Work out the finished part from the listing and answer in its coordinate system (mm). Face numbers are marked on the shaded views. Give positions to 0.01 mm unless a question says otherwise; leave off trailing zeros. Write each loop counter-clockwise with the first axis right and the second up, starting at its lowest first coordinate (ties: lowest second). Pieces come first, ordered by that corner, then holes. Notation, with made-up numbers: (77.5, 14) - (136.5, 14) arc R34 cw to (136.5, 47) - close; hole circle Ø5 at (-16.5, 5). An arc over 180 degrees is marked (long way). Write item = value, one per line.
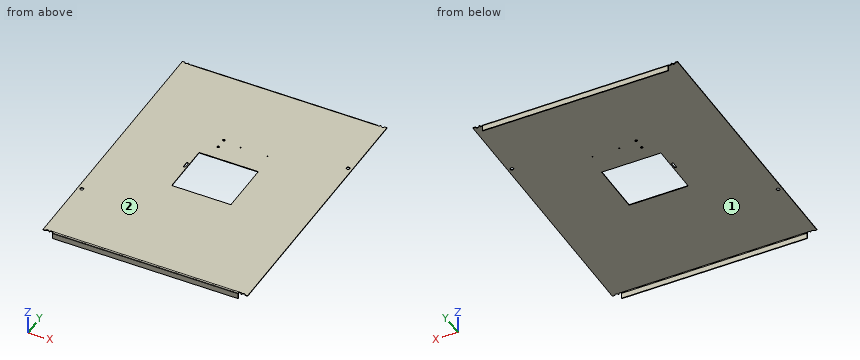
from build123d import *

# Parameters (mm, degrees)
CROQUIS1_W                   = 482.6
CROQUIS1_H                   = 634.238
BRIDA_BASE1_DEPTH            = 1.524
CROQUIS6_R                   = 3.9624
CROQUIS6_W                   = 6.35
CROQUIS6_H                   = 3.048
CORTAR_EXTRUIR1_DEPTH        = 399.487732229
BRIDA_START                  = -218.948
BRIDA_DE_ARISTA1_DEPTH       = 437.896
BRIDA_START_2                = -219.1004
BRIDA_DE_ARISTA1_2_OUTLINE_W = 0.1524
BRIDA_DE_ARISTA1_2_OUTLINE_H = 1.524
BRIDA_DE_ARISTA1_2_DEPTH     = 0.1524
BRIDA_START_3                = 218.948
BRIDA_DE_ARISTA1_3_OUTLINE_W = 0.1524
BRIDA_DE_ARISTA1_3_OUTLINE_H = 1.524
BRIDA_DE_ARISTA1_3_DEPTH     = 0.1524
BRIDA_DE_ARISTA1_4_DEPTH     = 437.896
CORTAR_EXTRUIR2_REACH        = 400.806
CROQUIS13_R                  = 3.9624
CROQUIS13_R_2                = 2.8956
CROQUIS13_R_3                = 1.27
CROQUIS13_W                  = 139.7
CROQUIS13_H                  = 124.714
CROQUIS13_W_2                = 4.826
CROQUIS13_H_2                = 16.002


# Read off the part's stored shape, not the designer's step: Brida de arista1
# Sheet-metal steps are written as plain solids
with BuildPart() as part:
    # Croquis1 → Brida base1 (new body)
    with BuildSketch(Plane.XY):
        Rectangle(CROQUIS1_W, CROQUIS1_H)
    extrude(amount=-BRIDA_BASE1_DEPTH)

    # Croquis6 → Cortar-Extruir1 (cut, through all)
    with BuildSketch(Plane.XY):
        with Locations((231.648, 317.627)):
            Circle(CROQUIS6_R)
        with Locations((-231.648, 317.627)):
            Circle(CROQUIS6_R)
        with Locations((-231.648, -317.627)):
            Circle(CROQUIS6_R)
        with Locations((231.648, -317.627)):
            Circle(CROQUIS6_R)
        with Locations((-222.123, 315.595)):
            Rectangle(CROQUIS6_W, CROQUIS6_H)
        with Locations((222.123, 315.595)):
            Rectangle(CROQUIS6_W, CROQUIS6_H)
        with Locations((-222.123, -315.595)):
            Rectangle(CROQUIS6_W, CROQUIS6_H)
        with Locations((222.123, -315.595)):
            Rectangle(CROQUIS6_W, CROQUIS6_H)
    extrude(amount=-CORTAR_EXTRUIR1_DEPTH, mode=Mode.SUBTRACT)

    # Brida de arista1 outline → Brida de arista1 (cut)
    with BuildSketch(Plane.YZ.offset(BRIDA_START)):
        with BuildLine():
            ThreePointArc((-316.710645431, -1.524), (-315.595, -0.408354569), (-314.071, 0))
            Line((-314.071, 0), (-317.119, 0))
            Line((-317.119, 0), (-317.119, -1.524))
            Line((-317.119, -1.524), (-316.710645431, -1.524))
        make_face()
        with BuildLine():
            Line((317.119, 0), (314.071, 0))
            ThreePointArc((314.071, 0), (315.595, -0.408354569), (316.710645431, -1.524))
            Line((316.710645431, -1.524), (317.119, -1.524))
            Line((317.119, -1.524), (317.119, 0))
        make_face()
    extrude(amount=BRIDA_DE_ARISTA1_DEPTH, mode=Mode.SUBTRACT)

    # Brida de arista1 2 outline → Brida de arista1 2 (cut)
    with BuildSketch(Plane.YZ.offset(BRIDA_START_2)):
        with Locations((-313.9948, -0.762)):
            Rectangle(BRIDA_DE_ARISTA1_2_OUTLINE_W, BRIDA_DE_ARISTA1_2_OUTLINE_H)
        with Locations((313.9948, -0.762)):
            Rectangle(BRIDA_DE_ARISTA1_2_OUTLINE_W, BRIDA_DE_ARISTA1_2_OUTLINE_H)
    extrude(amount=BRIDA_DE_ARISTA1_2_DEPTH, mode=Mode.SUBTRACT)

    # Brida de arista1 3 outline → Brida de arista1 3 (cut)
    with BuildSketch(Plane.YZ.offset(BRIDA_START_3)):
        with Locations((-313.9948, -0.762)):
            Rectangle(BRIDA_DE_ARISTA1_3_OUTLINE_W, BRIDA_DE_ARISTA1_3_OUTLINE_H)
        with Locations((313.9948, -0.762)):
            Rectangle(BRIDA_DE_ARISTA1_3_OUTLINE_W, BRIDA_DE_ARISTA1_3_OUTLINE_H)
    extrude(amount=BRIDA_DE_ARISTA1_3_DEPTH, mode=Mode.SUBTRACT)

    # Brida de arista1 4 outline → Brida de arista1 4 (add)
    with BuildSketch(Plane.YZ.offset(BRIDA_START)):
        with BuildLine():
            ThreePointArc((-315.595, -3.048), (-315.148630735, -1.970369265), (-314.071, -1.524))
            Line((-314.071, -1.524), (-316.710645431, -1.524))
            ThreePointArc((-316.710645431, -1.524), (-317.015141918, -2.259119551), (-317.119, -3.048))
            Line((-317.119, -3.048), (-317.119, -16.002))
            Line((-317.119, -16.002), (-315.595, -16.002))
            Line((-315.595, -16.002), (-315.595, -3.048))
        make_face()
        with BuildLine():
            Line((316.710645431, -1.524), (314.071, -1.524))
            ThreePointArc((314.071, -1.524), (315.148630735, -1.970369265), (315.595, -3.048))
            Line((315.595, -3.048), (315.595, -16.002))
            Line((315.595, -16.002), (317.119, -16.002))
            Line((317.119, -16.002), (317.119, -3.048))
            ThreePointArc((317.119, -3.048), (317.015141918, -2.259119551), (316.710645431, -1.524))
        make_face()
    extrude(amount=BRIDA_DE_ARISTA1_4_DEPTH)

    # Croquis13 → Cortar-Extruir2 (cut, up to next)
    with BuildSketch(Plane.XY, mode=Mode.PRIVATE) as cortar_extruir2_sk1:
        with Locations((-231.648, -158.877)):
            Circle(CROQUIS13_R)
    cortar_extruir2_tool1 = extrude(cortar_extruir2_sk1.sketch, amount=-CORTAR_EXTRUIR2_REACH, mode=Mode.PRIVATE) & part.part
    # Croquis13 → Cortar-Extruir2 (cut, up to next)
    with BuildSketch(Plane.XY, mode=Mode.PRIVATE) as cortar_extruir2_sk2:
        with Locations((231.648, 158.877)):
            Circle(CROQUIS13_R)
    cortar_extruir2_tool2 = extrude(cortar_extruir2_sk2.sketch, amount=-CORTAR_EXTRUIR2_REACH, mode=Mode.PRIVATE) & part.part
    # Croquis13 → Cortar-Extruir2 (cut, up to next)
    with BuildSketch(Plane.XY, mode=Mode.PRIVATE) as cortar_extruir2_sk3:
        with Locations((-42.8498, 97.409)):
            Circle(CROQUIS13_R_2)
    cortar_extruir2_tool3 = extrude(cortar_extruir2_sk3.sketch, amount=-CORTAR_EXTRUIR2_REACH, mode=Mode.PRIVATE) & part.part
    # Croquis13 → Cortar-Extruir2 (cut, up to next)
    with BuildSketch(Plane.XY, mode=Mode.PRIVATE) as cortar_extruir2_sk4:
        with Locations((-42.8498, 122.809)):
            Circle(CROQUIS13_R_2)
    cortar_extruir2_tool4 = extrude(cortar_extruir2_sk4.sketch, amount=-CORTAR_EXTRUIR2_REACH, mode=Mode.PRIVATE) & part.part
    # Croquis13 → Cortar-Extruir2 (cut, up to next)
    with BuildSketch(Plane.XY, mode=Mode.PRIVATE) as cortar_extruir2_sk5:
        with Locations((0, 116.967)):
            Circle(CROQUIS13_R_3)
    cortar_extruir2_tool5 = extrude(cortar_extruir2_sk5.sketch, amount=-CORTAR_EXTRUIR2_REACH, mode=Mode.PRIVATE) & part.part
    # Croquis13 → Cortar-Extruir2 (cut, up to next)
    with BuildSketch(Plane.XY, mode=Mode.PRIVATE) as cortar_extruir2_sk6:
        with Locations((63.5, 116.967)):
            Circle(CROQUIS13_R_3)
    cortar_extruir2_tool6 = extrude(cortar_extruir2_sk6.sketch, amount=-CORTAR_EXTRUIR2_REACH, mode=Mode.PRIVATE) & part.part
    # Croquis13 → Cortar-Extruir2 (cut, up to next)
    with BuildSketch(Plane.XY, mode=Mode.PRIVATE) as cortar_extruir2_sk7:
        Rectangle(CROQUIS13_W, CROQUIS13_H)
    cortar_extruir2_tool7 = extrude(cortar_extruir2_sk7.sketch, amount=-CORTAR_EXTRUIR2_REACH, mode=Mode.PRIVATE) & part.part
    # Croquis13 → Cortar-Extruir2 (cut, up to next)
    with BuildSketch(Plane.XY, mode=Mode.PRIVATE) as cortar_extruir2_sk8:
        with Locations((-75.057, 12.954)):
            Rectangle(CROQUIS13_W_2, CROQUIS13_H_2)
    cortar_extruir2_tool8 = extrude(cortar_extruir2_sk8.sketch, amount=-CORTAR_EXTRUIR2_REACH, mode=Mode.PRIVATE) & part.part
    add(cortar_extruir2_tool1.solids().sort_by_distance((-231.648, -158.877, 0))[0], mode=Mode.SUBTRACT)
    add(cortar_extruir2_tool2.solids().sort_by_distance((231.648, 158.877, 0))[0], mode=Mode.SUBTRACT)
    add(cortar_extruir2_tool3.solids().sort_by_distance((-42.8498, 97.409, 0))[0], mode=Mode.SUBTRACT)
    add(cortar_extruir2_tool4.solids().sort_by_distance((-42.8498, 122.809, 0))[0], mode=Mode.SUBTRACT)
    add(cortar_extruir2_tool5.solids().sort_by_distance((0, 116.967, 0))[0], mode=Mode.SUBTRACT)
    add(cortar_extruir2_tool6.solids().sort_by_distance((63.5, 116.967, 0))[0], mode=Mode.SUBTRACT)
    add(cortar_extruir2_tool7.solids().sort_by_distance((0, 0, 0))[0], mode=Mode.SUBTRACT)
    add(cortar_extruir2_tool8.solids().sort_by_distance((-75.057, 12.954, 0))[0], mode=Mode.SUBTRACT)


solid = part.part
1. Find section C-C, the plane y = -130.5. Give the vertices of the cut face in (x, z), then the cut area to 3 significant figures.
Solution:
outline = (-241.3, -1.52) - (241.3, -1.52) - (241.3, 0) - (-241.3, 0) - close
area = 735 mm^2
2. Straight lines are drawn through the part: line 1 (Y direction, x = 0, z = -0.4); line 2 (Y direction, x = 63.5, z = -0.45); line 3 (Y direction, x = -173, z = -6.5) (3 decimals). For each, find the intervals that lie inside material, in ascending order.
Solution:
line_1 = -315.58 to -62.36, 62.36 to 115.7, 118.24 to 315.58
line_2 = -315.66 to -62.36, 62.36 to 115.7, 118.24 to 315.66
line_3 = -317.119 to -315.595, 315.595 to 317.119
3. Given pin 1 (1.7 mm diameter, centred on x = 223, z = -0.5, fed in from +Y); pin 2 (1 mm diameter, centred on y = 315.5, z = -7, fed in from +X); pin 3 (0.5 mm diameter, centred on x = -17.5, z = -0.5, fed in from -Y), each flat-ended and moving along its own axis, determine where each tip first touches the part or whether it passes through.
Solution:
pin_1 = 314.07
pin_2 = 218.95
pin_3 = -316.07
4. Find section A-A, the plane z = -12.5. Give the vertices of the cut face in (x, y) (3 decimals), then the cut area to 3 significant figures.
Solution:
outline = (-218.948, -317.119) - (218.948, -317.119) - (218.948, -315.595) - (-218.948, -315.595) - close; (-218.948, 315.595) - (218.948, 315.595) - (218.948, 317.119) - (-218.948, 317.119) - close
area = 1,330 mm^2
5. For a pull along Y with two mould halves and no side action, classify the marked faces 1 and 2 as pulls with the +Y half, pulls with the -Y half, needs draft (parallel to the pull), parting line crosses it, or undercut.
Solution:
face_1 = undercut
face_2 = needs draft
6. Find section B-B, the plane x = -195. Give the vertices of the cut face in (y, z) (3 decimals), then the cut area to 3 significant figures.
Solution:
outline = (-317.119, -16.002) - (-315.595, -16.002) - (-315.595, -3.048) arc R1.524 cw to (-314.071, -1.524) - (314.071, -1.524) arc R1.524 cw to (315.595, -3.048) - (315.595, -16.002) - (317.119, -16.002) - (317.119, -3.048) arc R3.048 ccw to (314.071, 0) - (-314.071, 0) arc R3.048 ccw to (-317.119, -3.048) - close
area = 1,010 mm^2
